Check sheet for the modelled part. Datum: model origin and axes. Units: mm. A direction names the side the tool comes from. Coordinates: 2 decimals unless noted, no trailing zeros. Loops run counter-clockwise (first coordinate to the right, second up) from the corner with the lowest first, then second, coordinate; pieces in that order, holes last. Notation, with made-up numbers: (-39, 76.25) -> (4, 76.25) arc R28 ccw to (4, 109.25) -> close; hole circle Ø8 at (6, 0). An arc over 180 degrees is marked (long way). Use one line per item in the form item = value.
from build123d import *

# Parameters (mm, degrees)
F0_W      = 42
F0_H      = 42
F1_DEPTH  = 34
F2_R      = 1.834542
F3_DEPTH  = 5
F4_R      = 5.169646
F5_DEPTH  = 2
F6_R      = 1.823353
F7_DEPTH  = 7
F8_R      = 5.110436
F9_DEPTH  = 2
F10_R     = 1.842077
F11_DEPTH = 7
F12_R     = 5.194055
F13_DEPTH = 2


with BuildPart() as f1:
    # F0 (on Front) → F1 (new body)
    with BuildSketch(Plane.XZ):
        with Locations((21, 21)):
            Rectangle(F0_W, F0_H)
    extrude(amount=F1_DEPTH)

    # F2 (on face) → F3 (join)
    with BuildSketch(Plane.XZ):
        with Locations((21.093497, 21.097444)):
            Circle(F2_R)
    extrude(amount=-F3_DEPTH)

    # F4 (on face) → F5 (join)
    with BuildSketch(Plane(origin=(0, 5, 0), x_dir=(-1, 0, 0), z_dir=(0, 1, 0))):
        with Locations((-21.093497, 21.097444)):
            Circle(F4_R)
    extrude(amount=F5_DEPTH)

    # F6 (on face) → F7 (join)
    with BuildSketch(Plane(origin=(0, 5, 0), x_dir=(-1, 0, 0), z_dir=(0, 1, 0))):
        with Locations((-21.252004, 21.045802)):
            Circle(F6_R)
    extrude(amount=F7_DEPTH)

    # F8 (on face) → F9 (join)
    with BuildSketch(Plane(origin=(0, 12, 0), x_dir=(-1, 0, 0), z_dir=(0, 1, 0))):
        with Locations((-21.252004, 21.045802)):
            Circle(F8_R)
    extrude(amount=F9_DEPTH)

    # F10 (on face) → F11 (join)
    with BuildSketch(Plane(origin=(0, 12, 0), x_dir=(-1, 0, 0), z_dir=(0, 1, 0))):
        with Locations((-21.252004, 21.045802)):
            Circle(F10_R)
    extrude(amount=F11_DEPTH)

    # F12 (on face) → F13 (join)
    with BuildSketch(Plane(origin=(0, 19, 0), x_dir=(-1, 0, 0), z_dir=(0, 1, 0))):
        with Locations((-21.252004, 21.045802)):
            Circle(F12_R)
    extrude(amount=F13_DEPTH)


solid = f1.part
(1) Section check C-C, the plane x = 33. Record the boundary of the cut face in (y, z).
Established:
outline = (-34, 0) -> (0, 0) -> (0, 42) -> (-34, 42) -> close
(2) Section check A-A, the plane x = 18. Record the boundary of the cut face in (y, z).
Established:
outline = (-34, 0) -> (0, 0) -> (0, 42) -> (-34, 42) -> close; (5, 16.96) -> (7, 16.96) -> (7, 25.24) -> (5, 25.24) -> close; (12, 17.1) -> (14, 17.1) -> (14, 24.99) -> (12, 24.99) -> close; (19, 17) -> (21, 17) -> (21, 25.1) -> (19, 25.1) -> close
(3) Section check D-D, the plane y = 4. Record the boundary of the cut face in (x, z), plus the area to 3 significant figures.
Established:
outline = circle Ø3.67 at (21.09, 21.1)
area = 10.6 mm²
(4) Scan line: line 1 along Y through (x, z) = (35.5, 39.5). Record every from-to range of solid material in increasing order.
Established:
line_1 = -34 to 0
(5) Go/stop test with a flat-tipped pin: P1, Ø1, axis at x = 10.5, z = 19.5, coming from the +Y side. Record where the tip stops, or that it passes through.
Established:
P1 = 0
(6) Tool access check on faces 5 (the flat face through (21, 21, 21)), 6 (the cylindrical face through (18.46, 19.986, 25.425)), 7 (the flat face through (21, 12, 19)). Record the directions out of +Z, -Z, +X, -X, +Y, -Y that give a thin tool (end or side, any length) a straight path to the whole face; none if there is none.
Established:
face_5 = +Z, -Z, +X, -X, +Y
face_6 = +Y
face_7 = none
(7) Mould release check, pull along Y, two halves, no side actions. Record for faces 1 (the flat face through (21, 7, 19)), 2 (the flat face through (42, -17, 21)), 3 (the flat face through (21, -34, 21)), 4 (the flat face through (21, 19, 19)): +Y half, -Y half, draft (parallel to the pull), parting line (faces both ways), or undercut.
Established:
face_1 = undercut
face_2 = draft
face_3 = -Y half
face_4 = undercut
(8) Section check B-B, the plane z = 17. Record the boundary of the cut face in (x, y).
Established:
outline = (0, -34) -> (42, -34) -> (42, 0) -> (0, 0) -> close; (17.94, 5) -> (24.25, 5) -> (24.25, 7) -> (17.94, 7) -> close; (17.99, 19) -> (24.51, 19) -> (24.51, 21) -> (17.99, 21) -> close; (18.13, 12) -> (24.37, 12) -> (24.37, 14) -> (18.13, 14) -> close
